Check sheet for the modelled part. Datum: model origin and axes. Units: mm. A direction names the side the tool comes from. Coordinates: 2 decimals unless noted, no trailing zeros. Loops run counter-clockwise (first coordinate to the right, second up) from the corner with the lowest first, then second, coordinate; pieces in that order, holes last. Notation, with made-up numbers: (6, -13) -> (55, -13) arc R15 ccw to (55, -3) -> close; hole circle Ø9 at (78.25, 59.5). An arc over 180 degrees is marked (long way). Use CSV: the item, a comma, the result in double quotes. Start each with the question number.
1. Set-up check for faces 4 (the face through (-27.392, -6, 34)), 5 (the face through (-47.392, -6, 32)): record each of +Z, -Z, +X, -X, +Y, -Y from which the full face is reachable in a straight line by a thin tool's end or side.
2. Sectioned sample at B-B, the plane y = -10. Record the cut outline in (x, z), and give its area (3 significant figures).
3. Sectioned sample at A-A, the plane z = 33. Record the cut outline in (x, y).
4. Sectioned sample at C-C, the plane x = -32. Record the cut outline in (y, z), and give its area (3 significant figures).
5. Thickness scan on L1, parallel to X at y = -4.25, z = 36.5; L2, parallel to Z at x = -32.25, y = -8.5; L3, parallel to Z at x = -33, y = -10.75. Record the ranges inside material, lowest first.
6. Release check for a two-part mould opening along X. For faces 1 (the face through (-33, -6, 51.838)), 2 (the face through (-17.392, -6, 32)), 3 (the face through (-37.392, -6, 34)) record: pulls with the +X half, pulls with the -X half, needs draft (parallel to the pull), parting line crosses it, or undercut.
```python
from build123d import *

# Parameters (mm, degrees)
F0_W     = 30
F0_H     = 40
F1_DEPTH = 12


with BuildPart() as f1:
    # F0 (on Front) → F1 (new body)
    with BuildSketch(Plane.XZ):
        with Locations((-32.392114, 31.837786)):
            Rectangle(F0_W, F0_H)
        with BuildLine():
            ThreePointArc((-37.392114, 36.837786), (-32.392114, 41.837786), (-27.392114, 36.837786))
            Line((-27.392114, 36.837786), (-27.392114, 31.837786))
            ThreePointArc((-27.392114, 31.837786), (-32.392114, 26.837786), (-37.392114, 31.837786))
            Line((-37.392114, 31.837786), (-37.392114, 36.837786))
        make_face(mode=Mode.SUBTRACT)
    extrude(amount=F1_DEPTH)


solid = f1.part
```
Completed:
1,face 4,"+Y, -Y"
1,face 5,"+Z, -Z, -X, +Y, -Y"
2,outline,"(-47.39, 11.84) -> (-17.39, 11.84) -> (-17.39, 51.84) -> (-47.39, 51.84) -> close; hole (-37.39, 31.84) arc R5 ccw to (-27.39, 31.84) -> (-27.39, 36.84) arc R5 ccw to (-37.39, 36.84) -> close"
2,area,"1,070 mm²"
3,outline,"(-47.39, -12) -> (-37.39, -12) -> (-37.39, 0) -> (-47.39, 0) -> close; (-27.39, -12) -> (-17.39, -12) -> (-17.39, 0) -> (-27.39, 0) -> close"
4,outline,"(-12, 11.84) -> (0, 11.84) -> (0, 26.85) -> (-12, 26.85) -> close; (-12, 41.82) -> (0, 41.82) -> (0, 51.84) -> (-12, 51.84) -> close"
4,area,"300 mm²"
5,L1,"-47.39 to -37.39, -27.39 to -17.39"
5,L2,"11.84 to 26.84, 41.84 to 51.84"
5,L3,"11.84 to 26.87, 41.8 to 51.84"
6,face 1,"needs draft"
6,face 2,"pulls with the +X half"
6,face 3,"undercut"
